Autodesk Inventor part; units mm, degrees
ref_plane "YZ Plane" through (0, 0, 0) normal (1, 0, 0) x (0, 1, 0)
ref_plane "XZ Plane" through (0, 0, 0) normal (0, 1, 0) x (-1, 0, 0)
ref_plane "XY Plane" through (0, 0, 0) normal (0, 0, 1) x (1, 0, 0)
sketch "Skizze1" plane through (0, 0, 0) normal (0, 0, 1) x (1, 0, 0)
  line L0 (-44.8, 0) -> (44.8, 0)
  line L1 (44.8, 0) -> (44.8, 2.5)
  line L2 (44.8, 2.5) -> (40, 2.5)
  line L3 (40, 2.5) -> (40, 3.25)
  line L4 (40, 3.25) -> (-33.7, 3.25)
  line L5 (-33.7, 3.25) -> (-33.7, 2.5)
  line L6 (-33.7, 2.5) -> (-44.8, 2.5)
  line L7 (-44.8, 2.5) -> (-44.8, 0)
  line L8 (0, 3.9) -> (0, -0.65)
  line L9 (-39.8, 2.5) -> (-39.8, 0) construction
  point P0 (0, 0)
  dimension "d1" = 4.8
  dimension "d2" = 5
  dimension "d4" = 6.5
  dimension "d18" = 5
  dimension "d20" = 79.8
  dimension "d22" = 6.1
  dimension "d23" = 5
revolve "Umdrehung1" add sketch "Skizze1" angle 360 about axis through (-44.8, 0, 0) along (1, 0, 0)
chamfer "Fase2" distance 0.4 angle 15 1 edges at (-44.8, -2.5, 0) measured on face at (-41.1, 2.4919, -0.2012)
chamfer "Fase3" distance 0.4 angle 15 1 edges at (44.8, -2.5, 0) measured on face at (41.6, 2.4919, -0.2012)
properties part number "Dribblingwelle" material "Aluminium 6061"
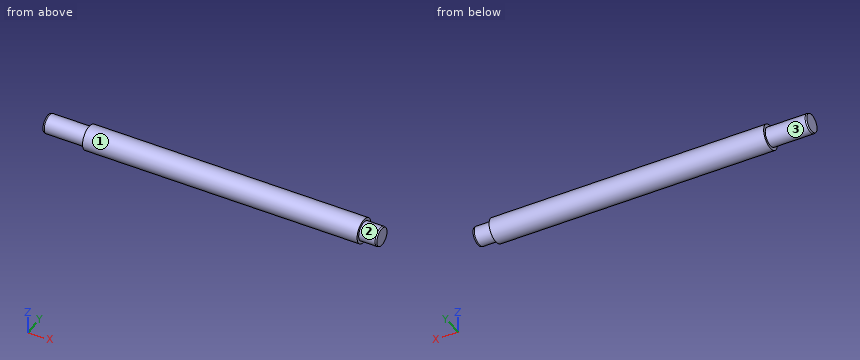
The listing builds one solid part. Answer for the finished solid, in the listing's coordinates (mm). Face numbers are marked on the shaded views. A direction names the side the tool comes from. Give positions to 0.01 mm unless a question says otherwise; leave off trailing zeros. Loops run counter-clockwise (first coordinate to the right, second up) from the corner with the lowest first, then second, coordinate; pieces in that order, holes last. Notation, with made-up numbers: M 12.25,67.25 L 57.25,67.25 A19 ccw 57.25,93.25 Z; hole C -22,-1 d11. An arc over 180 degrees is marked long. One line per item, written item: value.
1. Find the intervals of material crossed by probe 1 along X at (y, z) = (2.5, -1); probe 2 along Y at (x, z) = (-5, 0.25); probe 3 along Z at (x, y) = (-19, -2.5), in increasing order.
Found:
probe 1: -33.7 to 40
probe 2: -3.24 to 3.24
probe 3: -2.08 to 2.08
2. Section C-C on x = 18.5 is taken. Determine the outline of the cut face in (y, z).
Found:
outline: C 0,0 d6.5
3. This flat-tipped pin is pushed along its axis until it touches: P1, Ø2, axis at x = 18, y = -1.5, coming from the -Z side. Where does it stop, or does it pass through?
Found:
P1: z = -3.21
4. Section A-A on y = 0 is taken. Determine the outline of the cut face in (x, z).
Found:
outline: M -44.8,-2.39 L -44.4,-2.5 L -33.7,-2.5 L -33.7,-3.25 L 40,-3.25 L 40,-2.5 L 44.4,-2.5 L 44.8,-2.39 L 44.8,2.39 L 44.4,2.5 L 40,2.5 L 40,3.25 L -33.7,3.25 L -33.7,2.5 L -44.4,2.5 L -44.8,2.39 Z
5. For the marked faces 1, 2 and 3, determine the directions among +Z, -Z, +X, -X, +Y, -Y from which every point of the face is accessible in a straight line to the end or side of a thin tool.
Found:
face 1: +X, -X
face 2: +X
face 3: -X
